```python
from build123d import *

# Parameters (mm, degrees)
BOSS_EXTRUDE1_DEPTH      = 1.3843
BOSS_EXTRUDE1_DEPTH_BACK = 1.3843
SKETCH3_R                = 1.5875
CUT_EXTRUDE1_DEPTH       = 78.080989378


with BuildPart() as part:
    # Sketch3 → Boss-Extrude1 (new, two sides: drawn at the far end of the back side and taken through both)
    with BuildSketch(Plane.XY.offset(-BOSS_EXTRUDE1_DEPTH_BACK)):
        with BuildLine():
            Line((-13.67380138, -52.752331459), (-11.3157, -43.654982291))
            Line((-11.3157, -43.654982291), (-21.476062034, -39.655785263))
            ThreePointArc((-21.476062034, -39.655785263), (-24.823734092, -42.182520656), (-28.926434765, -41.311230152))
            ThreePointArc((-28.926434765, -41.311230152), (0, 46.3931), (28.926434765, -41.311230152))
            ThreePointArc((28.926434765, -41.311230152), (24.823734092, -42.182520656), (21.476062034, -39.655785263))
            Line((21.476062034, -39.655785263), (11.3157, -43.654982291))
            Line((11.3157, -43.654982291), (13.67380138, -52.752331459))
            ThreePointArc((13.67380138, -52.752331459), (0, 54.4957), (-13.67380138, -52.752331459))
        make_face()
        with Locations((-17.210160294, -43.724142128)):
            Circle(SKETCH3_R, mode=Mode.SUBTRACT)
        with Locations(Location((17.210160294, -43.724142128, 0), (0, 0, 180))):
            Circle(SKETCH3_R, mode=Mode.SUBTRACT)
    extrude(amount=BOSS_EXTRUDE1_DEPTH + BOSS_EXTRUDE1_DEPTH_BACK)

    # Sketch4 → Cut-Extrude1 (cut, symmetric)
    with BuildSketch(Plane.XY):
        with BuildLine():
            Line((-13.968711324, -52.675007569), (-13.968711324, -66.643718893))
            Line((-13.968711324, -66.643718893), (0, -66.643718893))
            Line((0, -66.643718893), (0, -54.4957))
            Line((0, -54.4957), (0, -43.561952925))
            Line((0, -43.561952925), (-11.552050454, -43.561952925))
            ThreePointArc((-11.552050454, -43.561952925), (-12.491783859, -48.189708607), (-13.968711324, -52.675007569))
        make_face()
    cut_extrude1 = extrude(amount=CUT_EXTRUDE1_DEPTH, both=True, mode=Mode.SUBTRACT)

    # Mirror1: Cut-Extrude1 across plane
    add(cut_extrude1.mirror(Plane(origin=(0, 0, 0), x_dir=(0, 0, 1), z_dir=(1, 0, 0))), mode=Mode.SUBTRACT)


solid = part.part
```
For this review, take the finished solid that the model builds, in its own axes (mm). A direction names the side the tool comes from. Coordinates: 2 decimals unless noted, no trailing zeros. Write each loop counter-clockwise with the first axis right and the second up, starting at its lowest first coordinate (ties: lowest second). Pieces come first, ordered by that corner, then holes. Notation, with made-up numbers: (-27, 87.5) - (-17, 87.5) arc R31 ccw to (-17, 112.5) - close; hole circle Ø11 at (42, -13.5). An arc over 180 degrees is marked (long way). Answer in a Markdown table with one row per item. Add a question column.
Q1. We need section D-D, the plane x = 0. State the section outline as (y, z) points, and give its area (3 significant figures).
Q2. We need section A-A, the plane x = -34.5. State the section outline as (y, z) points.
Q3. Draft analysis for pull direction X (two halves, no side actions). For faces 1 (the cylindrical face through (-12.475, -48.126, 0.019)), 2 (the cylindrical face through (-16.357, -42.386, -0.019)), 3 (the flat face through (-24, 41, -1.384)), 4 (the cylindrical face through (2.2, 54.45, -0.02)), state which applies: +X half, -X half, draft (parallel to the pull), parting line (faces both ways), or undercut.
Q4. For probe 1 along Y at (x, z) = (17, 0.25); probe 2 along Y at (x, z) = (0, 0.85); probe 3 along Y at (x, z) = (34.5, 0.95), list the stretches that pass through material, from the lowest coordinate up.
Q5. Tool access review of faces 5 (the flat face through (-24, 41, 1.384)), 6 (the flat face through (16.584, -41.582, -0.019)), 7 (the cylindrical face through (12.475, -48.126, 0.019)): name each direction out of +Z, -Z, +X, -X, +Y, -Y from which nothing blocks a thin tool from reaching the whole face with its end or side.
Q6. We need section B-B, the plane y = -6. State the section outline as (x, z) points.
Q7. We need section C-C, the plane z = 0.95. State the section outline as (x, y) points (1 decimal), and give its area (3 significant figures).
Answer list:
| question | item | result |
|---|---|---|
| 1 | outline | (46.39, -1.38) - (54.5, -1.38) - (54.5, 1.38) - (46.39, 1.38) - close |
| 1 | area | 22.4 mm2 |
| 2 | outline | (-42.18, -1.38) - (-36.49, -1.38) - (-36.49, 1.38) - (-42.18, 1.38) - close; (32.03, -1.38) - (42.18, -1.38) - (42.18, 1.38) - (32.03, 1.38) - close |
| 3 | face 1 | undercut |
| 3 | face 2 | undercut |
| 3 | face 3 | draft |
| 3 | face 4 | parting line |
| 4 | probe 1 | y = -51.78 to -45.3, -42.15 to -41.42, 43.32 to 51.78 |
| 4 | probe 2 | y = 46.39 to 54.5 |
| 4 | probe 3 | y = -42.18 to -36.49, 32.03 to 42.18 |
| 5 | face 5 | +Z, +X, -X, +Y, -Y |
| 5 | face 6 | +Z, -Z |
| 5 | face 7 | +Z, -Z, -Y |
| 6 | outline | (-54.16, -1.38) - (-48.48, -1.38) - (-48.48, 1.38) - (-54.16, 1.38) - close; (48.48, -1.38) - (54.16, -1.38) - (54.16, 1.38) - (48.48, 1.38) - close |
| 7 | outline | (-28.9, -41.3) arc R48.6 cw (long way) to (28.9, -41.3) arc R5.1 cw to (21.5, -39.7) - (11.6, -43.6) arc R40.1 ccw to (14, -52.7) arc R54.5 ccw (long way) to (-14, -52.7) arc R40.1 ccw to (-11.6, -43.6) - (-21.5, -39.7) arc R5.1 cw to start; hole circle Ø3.2 at (-17.2, -43.7); hole circle Ø3.2 at (17.2, -43.7) |
| 7 | area | 1,940 mm2 |
